```python
from build123d import *

# Parameters (mm, degrees)
SKETCH1_W           = 60
SKETCH1_H           = 40
BOSS_EXTRUDE1_DEPTH = 1.6
SKETCH2_W           = 23
SKETCH2_H           = 15
BOSS_EXTRUDE2_DEPTH = 25
SKETCH3_W           = 5
SKETCH3_H           = 8
BOSS_EXTRUDE3_DEPTH = 8
SKETCH4_R           = 1.651573935
SKETCH4_R_2         = 1.75
SKETCH4_R_3         = 1.546416864
BOSS_EXTRUDE4_DEPTH = 7
CUT_EXTRUDE1_REACH  = 45.875
SKETCH5_R           = 1.5


with BuildPart() as part:
    # Sketch1 → Boss-Extrude1 (new body)
    with BuildSketch(Plane(origin=(0, 0, 0), x_dir=(1, 0, 0), z_dir=(0, 1, 0))):
        Rectangle(SKETCH1_W, SKETCH1_H)
    extrude(amount=BOSS_EXTRUDE1_DEPTH)

    # Sketch2 → Boss-Extrude2 (add)
    with BuildSketch(Plane(origin=(0, 1.6, 0), x_dir=(1, 0, 0), z_dir=(0, 1, 0))):
        with Locations((-12.5, 9.746936541)):
            Rectangle(SKETCH2_W, SKETCH2_H)
        with Locations((12.5, 9.746936541)):
            Rectangle(SKETCH2_W, SKETCH2_H)
    extrude(amount=BOSS_EXTRUDE2_DEPTH)

    # Sketch3 → Boss-Extrude3 (add)
    with BuildSketch(Plane(origin=(0, 1.6, 0), x_dir=(1, 0, 0), z_dir=(0, 1, 0))):
        with Locations((-24.5, -11)):
            Rectangle(SKETCH3_W, SKETCH3_H)
        with Locations((24.5, -11)):
            Rectangle(SKETCH3_W, SKETCH3_H)
    extrude(amount=BOSS_EXTRUDE3_DEPTH)

    # Sketch4 → Boss-Extrude4 (add)
    with BuildSketch(Plane(origin=(0, 1.6, 0), x_dir=(1, 0, 0), z_dir=(0, 1, 0))):
        with Locations(Location((-14.609598895, -1.534440121, 0), (0, 0, 90))):
            Circle(SKETCH4_R)
        with Locations(Location((6.959010124, -3.998189047, 0), (0, 0, 90))):
            Circle(SKETCH4_R_2)
        with Locations(Location((-12.405191961, -10.87075184, 0), (0, 0, 90))):
            Circle(SKETCH4_R_3)
        with Locations(Location((12.923875945, -3.998189047, 0), (0, 0, 90))):
            Circle(SKETCH4_R_2)
    extrude(amount=BOSS_EXTRUDE4_DEPTH)

    # Sketch5 → Cut-Extrude1 (cut, up to next)
    with BuildSketch(Plane(origin=(0, 1.6, 0), x_dir=(1, 0, 0), z_dir=(0, 1, 0)), mode=Mode.PRIVATE) as cut_extrude1_sk1:
        with Locations(Location((-27, 17, 0), (0, 0, 270))):
            Circle(SKETCH5_R)
    cut_extrude1_tool1 = extrude(cut_extrude1_sk1.sketch, amount=-CUT_EXTRUDE1_REACH, mode=Mode.PRIVATE) & part.part
    # Sketch5 → Cut-Extrude1 (cut, up to next)
    with BuildSketch(Plane(origin=(0, 1.6, 0), x_dir=(1, 0, 0), z_dir=(0, 1, 0)), mode=Mode.PRIVATE) as cut_extrude1_sk2:
        with Locations(Location((-27, -17, 0), (0, 0, 270))):
            Circle(SKETCH5_R)
    cut_extrude1_tool2 = extrude(cut_extrude1_sk2.sketch, amount=-CUT_EXTRUDE1_REACH, mode=Mode.PRIVATE) & part.part
    # Sketch5 → Cut-Extrude1 (cut, up to next)
    with BuildSketch(Plane(origin=(0, 1.6, 0), x_dir=(1, 0, 0), z_dir=(0, 1, 0)), mode=Mode.PRIVATE) as cut_extrude1_sk3:
        with Locations(Location((27, -17, 0), (0, 0, 270))):
            Circle(SKETCH5_R)
    cut_extrude1_tool3 = extrude(cut_extrude1_sk3.sketch, amount=-CUT_EXTRUDE1_REACH, mode=Mode.PRIVATE) & part.part
    # Sketch5 → Cut-Extrude1 (cut, up to next)
    with BuildSketch(Plane(origin=(0, 1.6, 0), x_dir=(1, 0, 0), z_dir=(0, 1, 0)), mode=Mode.PRIVATE) as cut_extrude1_sk4:
        with Locations(Location((27, 17, 0), (0, 0, 270))):
            Circle(SKETCH5_R)
    cut_extrude1_tool4 = extrude(cut_extrude1_sk4.sketch, amount=-CUT_EXTRUDE1_REACH, mode=Mode.PRIVATE) & part.part
    add(cut_extrude1_tool1.solids().sort_by_distance((-27, 1.6, -17))[0], mode=Mode.SUBTRACT)
    add(cut_extrude1_tool2.solids().sort_by_distance((-27, 1.6, 17))[0], mode=Mode.SUBTRACT)
    add(cut_extrude1_tool3.solids().sort_by_distance((27, 1.6, 17))[0], mode=Mode.SUBTRACT)
    add(cut_extrude1_tool4.solids().sort_by_distance((27, 1.6, -17))[0], mode=Mode.SUBTRACT)


solid = part.part
```
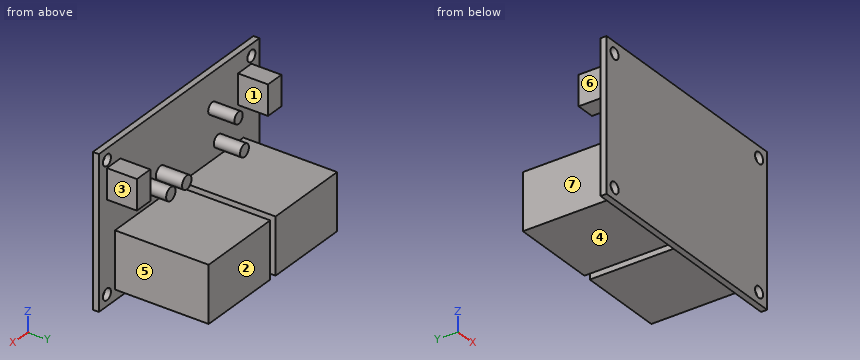
Could you check a few things on this model? Use its own coordinates, in mm. Face numbers are marked on the shaded views. A direction names the side the tool comes from. Coordinates: 2 decimals unless noted, no trailing zeros. Order: outer loops, then holes, each group sorted by start corner. A loop starts at its lowest first (then second) coordinate and runs counter-clockwise, first axis right, second up. Notation, with made-up numbers: M -10.5,58 L 44.5,58 A23 cw 44.5,84 Z; hole C -16,23 d10. An arc over 180 degrees is marked long. Use a Markdown table: item, result. Add a question column.
Q1. If I drill on L1, parallel to X at y = 1.3, z = 17; L2, parallel to X at y = 5.25, z = 8.5; L3, parallel to X at y = 21, z = -9, over which ranges is the centre line in solid material (lowest first)?
Q2. Which directions (+Z, -Z, +X, -X, +Y, -Y) give clear straight access to the entire face, cutting with the end or side of a thin tool? Please do the marked faces 4, 5, 6 and 7.
Q3. I want a section at C-C on x = -2.5. List the corners of the cut face in (y, z) for me.
Q4. We'd pull the mould along X, two halves only. Please class the marked faces 1, 2 and 3: pulls with the +X half, pulls with the -X half, needs draft (parallel to the pull), parting line crosses it, or undercut.
Q5. I'm going to push flat-ended pins straight in: pin 1 (1.5 mm diameter, centred on x = -24, z = 13, fed in from +Y); pin 2 (5 mm diameter, centred on x = -16.5, y = 18.5, fed in from +Z); pin 3 (2 mm diameter, centred on x = 6.5, z = 15.5, fed in from +Y); pin 4 (1.8 mm diameter, centred on x = -27, z = -17, fed in from +Y). Where does each tip first touch, or does it pass through?
Q6. I want a section at B-B on y = 13.25. List the corners of the cut face in (x, z) for me, then the cut area to 3 significant figures.
Q7. I want a section at A-A on z = 17. List the corners of the cut face in (x, y) for me.
Q8. I want a section at D-D on y = 6.75. List the corners of the cut face in (x, z) for me.
Checked values:
| question | item | result |
|---|---|---|
| 1 | L1 | -30 to -28.5, -25.5 to 25.5, 28.5 to 30 |
| 1 | L2 | -27 to -22, 22 to 27 |
| 1 | L3 | -24 to -1, 1 to 24 |
| 2 | face 4 | -Z, +X, -X, +Y |
| 2 | face 5 | -Z, +X, +Y |
| 2 | face 6 | +Z, -Z, -X, +Y |
| 2 | face 7 | -Z, -X, +Y |
| 3 | outline | M 0,-20 L 1.6,-20 L 1.6,-17.25 L 26.6,-17.25 L 26.6,-2.25 L 1.6,-2.25 L 1.6,20 L 0,20 Z |
| 4 | face 1 | undercut |
| 4 | face 2 | needs draft |
| 4 | face 3 | pulls with the +X half |
| 5 | pin 1 | y = 9.6 |
| 5 | pin 2 | z = -2.25 |
| 5 | pin 3 | y = 1.6 |
| 5 | pin 4 | through |
| 6 | outline | M -24,-17.25 L -1,-17.25 L -1,-2.25 L -24,-2.25 Z; M 1,-17.25 L 24,-17.25 L 24,-2.25 L 1,-2.25 Z |
| 6 | area | 690 mm² |
| 7 | outline | M -30,0 L -28.5,0 L -28.5,1.6 L -30,1.6 Z; M -25.5,0 L 25.5,0 L 25.5,1.6 L -25.5,1.6 Z; M 28.5,0 L 30,0 L 30,1.6 L 28.5,1.6 Z |
| 8 | outline | M -27,7 L -22,7 L -22,15 L -27,15 Z; M -24,-17.25 L -1,-17.25 L -1,-2.25 L -24,-2.25 Z; C -14.61,1.53 d3.3; C -12.41,10.87 d3.09; M 1,-17.25 L 24,-17.25 L 24,-2.25 L 1,-2.25 Z; C 6.96,4 d3.5; C 12.92,4 d3.5; M 22,7 L 27,7 L 27,15 L 22,15 Z |
